Could you check a few things on this model? Use its own coordinates, in mm. A direction names the side the tool comes from. Coordinates: 2 decimals unless noted, no trailing zeros. Write each loop counter-clockwise with the first axis right and the second up, starting at its lowest first coordinate (ties: lowest second). Pieces come first, ordered by that corner, then holes.
```python
from build123d import *

# Parameters (mm, degrees)
EXTRUDE_1_DEPTH          = 4
EXTRUDE_1_DEPTH_BACK     = 19
SKETCH_2_W               = 15.2
SKETCH_2_H               = 15.221861726
CUT_EXTRUDE_1_DEPTH      = 67
CUT_EXTRUDE_2_DEPTH      = 67
CUT_EXTRUDE_2_DEPTH_BACK = 67
SKETCH_3_R               = 2.15
SKETCH_4_R               = 4
CUT_EXTRUDE_3_DEPTH      = 67
SKETCH_5_R               = 2.15
CUT_EXTRUDE_4_DEPTH      = 67


with BuildPart() as part:
    # Sketch 1 → Extrude 1 (new, two sides: drawn at the far end of the back side and taken through both)
    with BuildSketch(Plane.XY.offset(-EXTRUDE_1_DEPTH_BACK)):
        Polygon((-23, 312.827661494), (-23, 297.827661494), (-38, 297.827661494), (-38, 293.827661494), (-30.870057685, 293.827661494), (-13.899494937, 276.857098745), (-11.071067812, 279.68552587), (-0.464466094, 290.292127588), align=None)
    extrude(amount=EXTRUDE_1_DEPTH + EXTRUDE_1_DEPTH_BACK)

    # Sketch 2 → Cut-Extrude 1 (cut)
    with BuildSketch(Plane(origin=(-145.378296841, 145.378296841, 0), x_dir=(0, 0, -1), z_dir=(0.7071067811865483, -0.7071067811865468, 0))):
        with Locations((7.5, 197.450035681)):
            Rectangle(SKETCH_2_W, SKETCH_2_H)
    extrude(amount=-CUT_EXTRUDE_1_DEPTH, mode=Mode.SUBTRACT)

    # Sketch 3 → Cut-Extrude 2 (cut, two sides: drawn at the far end of the back side and taken through both)
    with BuildSketch(Plane.XZ.offset(-293.827661494).offset(-CUT_EXTRUDE_2_DEPTH_BACK)):
        with Locations(Location((-32, -2, 0), (0, 0, 90))):
            Circle(SKETCH_3_R)
        with Locations(Location((-32, -13, 0), (0, 0, 90))):
            Circle(SKETCH_3_R)
    extrude(amount=CUT_EXTRUDE_2_DEPTH + CUT_EXTRUDE_2_DEPTH_BACK, mode=Mode.SUBTRACT)

    # Sketch 4 → Cut-Extrude 3 (cut)
    with BuildSketch(Plane.XZ.offset(-293.827661494)):
        with Locations((-32, -2)):
            Circle(SKETCH_4_R)
        with Locations((-32, -13)):
            Circle(SKETCH_4_R)
    extrude(amount=CUT_EXTRUDE_3_DEPTH, mode=Mode.SUBTRACT)

    # Sketch 5 → Cut-Extrude 4 (cut)
    with BuildSketch(Plane(origin=(131.478801904, 131.478801904, 0), x_dir=(0, 0, 1), z_dir=(-0.7071067811865472, -0.7071067811865478, 0))):
        with Locations(Location((-7.5, 213.595959067, 0), (0, 0, 270))):
            Circle(SKETCH_5_R)
    extrude(amount=-CUT_EXTRUDE_4_DEPTH, mode=Mode.SUBTRACT)


solid = part.part
```
Item 1: Which directions (+Z, -Z, +X, -X, +Y, -Y) give clear straight access to the entire face, cutting with the end or side of a thin tool? Please do faces 1 (the flat face through (-23, 305, -17)), 2 (the cylindrical face through (-28, 293, -2)), 3 (the flat face through (-14, 293, 0.1)).
Item 2: Will these pins go through, and if not, where does the flat tip stop? pin 1 Ø4.5 at (y, z) = (306.5, -16.5) entering from -X; pin 2 Ø4.5 at (x, z) = (-33, -4.5) entering from +Y; pin 3 Ø12 at (y, z) = (308, -4) entering from +X; pin 4 Ø10 at (x, z) = (-4.5, -8) entering from -Y.
Item 3: I want a section at B-B, the plane z = -13. List the corners of the cut face in (x, y) for me, then the cut area to 3 significant figures.
Item 4: I want a section at A-A, the plane x = -32. List the corners of the cut face in (y, z) for me, then the cut area to 3 significant figures.
Item 5: I want a section at D-D, the plane y = 293. List the corners of the cut face in (x, z) for me.
Item 6: I want a section at C-C, the plane y = 301.5. List the corners of the cut face in (x, z) for me, then the cut area to 3 significant figures.
Item 7: If we mould it in two halves opening along Y, with no side actions, what happens to faces 4 (the flat face through (-20.121, 288.594, -7.394)), 5 (the flat face through (-38, 296, -8)), 6 (the cylindrical face through (-19.72, 285.39, -7.41)), 7 (the flat face through (-34, 293.828, -8))? For each: released by +Y, released by -Y, zero draft, split by the parting line, or undercut.
Item 8: If I drill on line 1 along Y through (x, z) = (-34, -9.25); line 2 along Z through (x, y) = (-20, 296.5); line 3 along X through (y, z) = (296.35, -2), over which ranges is the centre line in solid material (lowest first)?
Taken from the geometry:
1. face 1: +Z, -Z, -X, +Y
1. face 2: -X, -Y
1. face 3: +X, +Y
2. pin 1: stops at x = -23
2. pin 2: stops at y = 297.83
2. pin 3: stops at x = -13.79
2. pin 4: passes through
3. outline: (-38, 293.83) - (-34.15, 293.83) - (-34.15, 297.83) - (-38, 297.83) - close; (-29.85, 293.83) - (-28, 293.83) - (-28, 290.96) - (-13.9, 276.86) - (-11.14, 279.61) - (-29.35, 297.83) - (-29.85, 297.83) - close
3. area: 107 mm2
4. outline: (293.83, -19) - (297.83, -19) - (297.83, -15.15) - (293.83, -15.15) - close; (293.83, -10.85) - (297.83, -10.85) - (297.83, -4.15) - (293.83, -4.15) - close; (293.83, 0.15) - (297.83, 0.15) - (297.83, 4) - (293.83, 4) - close
4. area: 57.6 mm2
5. outline: (-30.04, -19) - (-3.17, -19) - (-3.17, -15.1) - (-24.53, -15.1) - (-24.53, 0.1) - (-3.17, 0.1) - (-3.17, 4) - (-30.04, 4) - (-30.04, 1.49) arc R4 cw to (-30.04, -5.49) - (-30.04, -9.51) arc R4 cw to (-30.04, -16.49) - close
6. outline: (-23, -19) - (-11.67, -19) - (-11.67, -15.1) - (-23, -15.1) - close; (-23, 0.1) - (-11.67, 0.1) - (-11.67, 4) - (-23, 4) - close
6. area: 88.4 mm2
7. face 4: released by +Y
7. face 5: zero draft
7. face 6: undercut
7. face 7: released by -Y
8. line 1: y = 293.83 to 297.83
8. line 2: z = -19 to -15.1, 0.1 to 4
8. line 3: x = -38 to -34.15, -29.85 to -27.88
